```python
from build123d import *

# Parameters (mm, degrees)
SKETCH1_W           = 85.87
SKETCH1_H           = 66
BOSS_EXTRUDE2_DEPTH = 5
FILLET1_R           = 5
CUT_EXTRUDE2_DEPTH  = 3
CUT_EXTRUDE1_REACH  = 7
SKETCH2_W           = 57.29
SKETCH2_H           = 38.19
FILLET2_R           = 3
SKETCH3_R           = 1.5
BOSS_EXTRUDE3_DEPTH = 3


with BuildPart() as part:
    # Sketch1 → Boss-Extrude2 (new body)
    with BuildSketch(Plane.XY):
        with Locations((39.935, 30)):
            Rectangle(SKETCH1_W, SKETCH1_H)
    extrude(amount=BOSS_EXTRUDE2_DEPTH)

    # Fillet1
    fillet1_edges = [part.edges().sort_by_distance(p)[0] for p in [
        (82.87, -3, 2.5),
        (-3, -3, 2.5),
    ]]
    fillet(fillet1_edges, radius=FILLET1_R)

    # Sketch4 → Cut-Extrude2 (cut)
    with BuildSketch(Plane(origin=(0, 0, 0), x_dir=(-1, 0, 0), z_dir=(0, 0, -1))):
        with BuildLine():
            Line((-80.87, 61), (-80.87, 2))
            ThreePointArc((-80.87, 2), (-79.991320344, -0.121320344), (-77.87, -1))
            Line((-77.87, -1), (-2, -1))
            ThreePointArc((-2, -1), (0.121320344, -0.121320344), (1, 2))
            Line((1, 2), (1, 61))
            Line((1, 61), (-80.87, 61))
        make_face()
    extrude(amount=-CUT_EXTRUDE2_DEPTH, mode=Mode.SUBTRACT)

    # Sketch2 → Cut-Extrude1 (cut, up to next)
    with BuildSketch(Plane.XY.offset(5), mode=Mode.PRIVATE) as cut_extrude1_sk1:
        with Locations((39.935, 30)):
            Rectangle(SKETCH2_W, SKETCH2_H)
    cut_extrude1_tool1 = extrude(cut_extrude1_sk1.sketch, amount=-CUT_EXTRUDE1_REACH, mode=Mode.PRIVATE) & part.part
    add(cut_extrude1_tool1.solids().sort_by_distance((39.935, 30, 5))[0], mode=Mode.SUBTRACT)

    # Fillet2
    fillet2_edges = [part.edges().sort_by_distance(p)[0] for p in [
        (11.29, 10.905, 4),
        (11.29, 49.095, 4),
        (68.58, 49.095, 4),
        (68.58, 10.905, 4),
    ]]
    fillet(fillet2_edges, radius=FILLET2_R)

    # Sketch3 → Boss-Extrude3 (add)
    with BuildSketch(Plane(origin=(0, 0, 3), x_dir=(-1, 0, 0), z_dir=(0, 0, -1))):
        with Locations((-4, 4)):
            Circle(SKETCH3_R)
        with Locations((-4, 56)):
            Circle(SKETCH3_R)
        with Locations((-70.3, 56)):
            Circle(SKETCH3_R)
        with Locations((-70.3, 4)):
            Circle(SKETCH3_R)
    extrude(amount=BOSS_EXTRUDE3_DEPTH)


solid = part.part
```
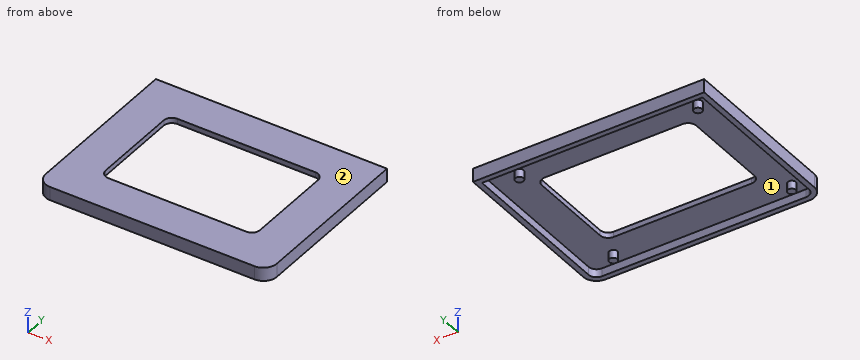
The listing builds one solid part. Answer for the finished solid, in the listing's coordinates (mm). Face numbers are marked on the shaded views. Give positions to 0.01 mm unless a question says otherwise; leave off trailing zeros. Write each loop counter-clockwise with the first axis right and the second up, starting at its lowest first coordinate (ties: lowest second). Pieces come first, ordered by that corner, then holes. Notation, with made-up numbers: (46.5, 64) -> (101.5, 64) arc R12 ccw to (101.5, 84) -> close; hole circle Ø3 at (35.5, -10.75). An arc over 180 degrees is marked (long way). Write item = value, one per line. Start each with the question number.
1) The part is cut by section A-A, the plane z = 1.7. Determine the outline of the cut face in (x, y), and give its area (3 significant figures).
2) The part is cut by section D-D, the plane x = 4. Determine the outline of the cut face in (y, z).
3) Straight lines are drawn through the part: line 1 along X through (y, z) = (20.5, 3.85); line 2 along X through (y, z) = (59.5, 1.4); line 3 along Y through (x, z) = (7.5, 0.75). For each, find the intervals that lie inside material, in ascending order.
4) The part is cut by section B-B, the plane x = 37. Determine the outline of the cut face in (y, z) (3 decimals), and give its area (3 significant figures).
5) The part is cut by section C-C, the plane y = 45. Determine the outline of the cut face in (x, z).
6) Determine the mould class of the marked faces 1 and 2 for opening direction Y: +Y half, -Y half, draft (parallel to the pull), parting line (faces both ways), or undercut.
Solutions:
q1.outline = (-3, 2) arc R5 ccw to (2, -3) -> (77.87, -3) arc R5 ccw to (82.87, 2) -> (82.87, 63) -> (-3, 63) -> close; circle Ø3 at (4, 4); circle Ø3 at (4, 56); circle Ø3 at (70.3, 4); circle Ø3 at (70.3, 56); hole (-1, 2) arc R3 ccw to (2, -1) -> (77.87, -1) arc R3 ccw to (80.87, 2) -> (80.87, 61) -> (-1, 61) -> close
q1.area = 613 mm²
q2.outline = (-3, 0) -> (-1, 0) -> (-1, 3) -> (2.5, 3) -> (2.5, 0) -> (5.5, 0) -> (5.5, 3) -> (54.5, 3) -> (54.5, 0) -> (57.5, 0) -> (57.5, 3) -> (61, 3) -> (61, 0) -> (63, 0) -> (63, 5) -> (-3, 5) -> close
q3.line_1 = -3 to 11.29, 68.58 to 82.87
q3.line_2 = -3 to -1, 80.87 to 82.87
q3.line_3 = -3 to -1, 61 to 63
q4.outline = (-3, 0) -> (-1, 0) -> (-1, 3) -> (10.905, 3) -> (10.905, 5) -> (-3, 5) -> close; (49.095, 3) -> (61, 3) -> (61, 0) -> (63, 0) -> (63, 5) -> (49.095, 5) -> close
q4.area = 67.6 mm²
q5.outline = (-3, 0) -> (-1, 0) -> (-1, 3) -> (11.29, 3) -> (11.29, 5) -> (-3, 5) -> close; (68.58, 3) -> (80.87, 3) -> (80.87, 0) -> (82.87, 0) -> (82.87, 5) -> (68.58, 5) -> close
q6.face_1 = undercut
q6.face_2 = draft
